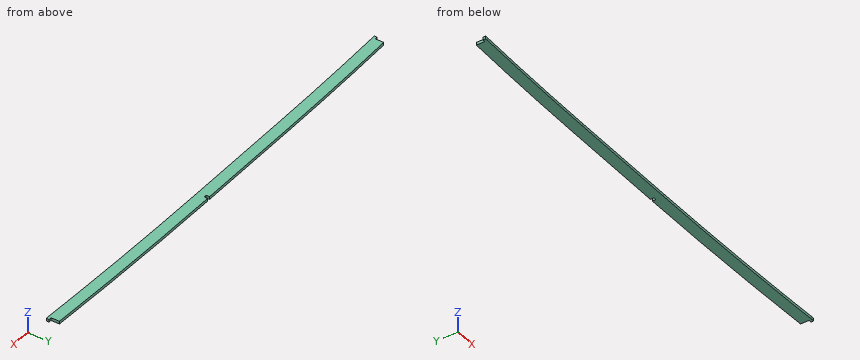
from build123d import *

# Parameters (mm, degrees)
BOSS_EXTRUDE1_DEPTH = 10


with BuildPart() as part:
    # Sketch1 → Boss-Extrude1 (new body)
    with BuildSketch(Plane.XY):
        with BuildLine():
            Line((-70.170888572, 381.474129778), (-477.5, 381.474129778))
            ThreePointArc((-477.5, 381.474129778), (-727.537146474, 379.319055722), (-977.5, 372.854473884))
            Line((-977.5, 372.854473884), (-977.5, 342.830625486))
            Line((-977.5, 342.830625486), (-987.5, 342.830625486))
            Line((-987.5, 342.830625486), (-987.5, 332.830625486))
            Line((-987.5, 332.830625486), (-977.5, 332.830625486))
            ThreePointArc((-977.5, 332.830625486), (-727.537352293, 339.31309229), (-477.5, 341.474129778))
            Line((-477.5, 341.474129778), (-60.170888572, 341.474129778))
            ThreePointArc((-60.170888572, 341.474129778), (237.427772245, 338.863423493), (534.934829654, 331.032108233))
            ThreePointArc((534.934829654, 331.032108233), (606.852618205, 328.354762156), (678.758400695, 325.372324122))
            Line((678.758400695, 325.372324122), (688.758400695, 325.372324122))
            Line((688.758400695, 325.372324122), (688.758400695, 335.372324122))
            Line((688.758400695, 335.372324122), (678.758400695, 335.372324122))
            Line((678.758400695, 335.372324122), (678.758400695, 365.410239494))
            ThreePointArc((678.758400695, 365.410239494), (309.381050642, 377.45768283), (-60.170888572, 381.474129778))
            Line((-60.170888572, 381.474129778), (-60.170888572, 368.974129778))
            Line((-60.170888572, 368.974129778), (-70.170888572, 368.974129778))
            Line((-70.170888572, 368.974129778), (-70.170888572, 381.474129778))
        make_face()
    extrude(amount=BOSS_EXTRUDE1_DEPTH)


solid = part.part
Check sheet for the modelled part. Datum: model origin and axes. Units: mm. Round coordinates to 2 decimals unless told otherwise and drop trailing zeros. Loops run counter-clockwise (first coordinate to the right, second up) from the corner with the lowest first, then second, coordinate; pieces in that order, holes last.
1. Sectioned sample at A-A on z = 5.5. Record the boundary of the cut face in (x, y), and give its area (3 significant figures).
2. Scan lines: probe 1 along X at (y, z) = (365, 5.25); probe 2 along Y at (x, z) = (-94.5, 9.25); probe 3 along Y at (x, z) = (-752, 6.25). Record each from-to range of solid material in increasing order.
3. Sectioned sample at C-C on x = 113.5. Record the boundary of the cut face in (y, z), and give its area (3 significant figures).
4. Gauge pin test, flat ends, axial feed: pin 1 Ø2 at (y, z) = (352.5, 6.5) entering from +X; pin 2 Ø5 at (x, z) = (-67, 7) entering from +Y; pin 3 Ø8 at (x, y) = (-160, 375) entering from -Z; pin 4 Ø3 at (x, z) = (-230, 7) entering from -Y. Record the tip position at first contact, or that the pin passes through.
5. Sectioned sample at B-B on x = -362.5. Record the boundary of the cut face in (y, z), and give its area (3 significant figures).
Recorded:
1. outline: (-987.5, 332.83) - (-977.5, 332.83) arc R14466.05 cw to (-477.5, 341.47) - (-60.17, 341.47) arc R16963.18 cw to (534.93, 331.03) arc R16963.18 cw to (678.76, 325.37) - (688.76, 325.37) - (688.76, 335.37) - (678.76, 335.37) - (678.76, 365.41) arc R17003.18 ccw to (-60.17, 381.47) - (-60.17, 368.97) - (-70.17, 368.97) - (-70.17, 381.47) - (-477.5, 381.47) arc R14506.05 ccw to (-977.5, 372.85) - (-977.5, 342.83) - (-987.5, 342.83) - close
1. area: 66,300 mm2
2. probe 1: x = -977.5 to 678.76
2. probe 2: y = 341.47 to 381.47
2. probe 3: y = 338.87 to 378.88
3. outline: (340.59, 0) - (380.59, 0) - (380.59, 10) - (340.59, 10) - close
3. area: 400 mm2
4. pin 1: stops at x = 678.76
4. pin 2: stops at y = 368.97
4. pin 3: stops at z = 0
4. pin 4: stops at y = 341.47
5. outline: (341.47, 0) - (381.47, 0) - (381.47, 10) - (341.47, 10) - close
5. area: 400 mm2
